Autodesk Inventor part; units mm, degrees
ref_plane "YZ Plane" through (0, 0, 0) normal (1, 0, 0) x (0, 1, 0)
ref_plane "XZ Plane" through (0, 0, 0) normal (0, 1, 0) x (-1, 0, 0)
ref_plane "XY Plane" through (0, 0, 0) normal (0, 0, 1) x (1, 0, 0)
sketch "Sketch1" plane through (0, 0, 0) normal (0, 1, 0) x (-1, 0, 0)
  line L0 (30, 30) -> (-30, 30)
  line L1 (-30, 30) -> (-30, -30)
  line L2 (-30, -30) -> (30, -30)
  line L3 (30, -30) -> (30, 30)
  line L4 (30, 30) -> (-30, -30) construction
  line L5 (-30, 30) -> (30, -30) construction
  circle A0 centre (0, 0) radius 29
  circle A1 centre (0, 0) radius 30
  point P0 (0, 0)
  dimension "d0" = 60
  dimension "d1" = 60
  dimension "d2" = 58
extrude "Extrusion1" add sketch "Sketch1" along normal blind 28 contours L3 A1 L0 | A1 L1 L0 | A1 | L3 L2 A1 | A1 L2 L1 | A0
sketch "Sketch2" plane through (0, 28, 0) normal (0, 1, 0) x (1, 0, 0)
  circle A0 centre (0, 0) radius 30
extrude "Extrusion2" add sketch "Sketch2" along normal blind 3
sketch "Sketch3" plane through (0, 31, 0) normal (0, 1, 0) x (1, 0, 0)
  circle A0 centre (0, 0) radius 29
  dimension "d7" = 58
extrude "Extrusion3" add sketch "Sketch3" along normal blind 39.5
sketch "Sketch4" plane through (0, 70.5, 0) normal (0, 1, 0) x (1, 0, 0)
  line L0 (-30, -30) -> (30, -30)
  line L1 (30, -30) -> (30, 30)
  line L2 (-30, -30) -> (30, -30)
  line L3 (30, -30) -> (30, 30)
  line L4 (30, 30) -> (-30, 30)
  line L5 (-30, 30) -> (-30, -30)
  line L6 (30, 30) -> (-30, 30) construction
  line L7 (-30, -30) -> (30, 30) construction
  line L8 (30, -30) -> (-30, 30) construction
  circle A0 centre (-23.575, -23.575) radius 2.5
  circle A1 centre (-23.575, 23.575) radius 2.5
  circle A2 centre (23.575, 23.575) radius 2.5
  circle A3 centre (23.575, -23.575) radius 2.5
  line L9 (-23.575, -23.575) -> (-23.575, 23.575) construction
  point P0 (0, 0)
  dimension "d10" = 5
  dimension "d11" = 5
  dimension "d12" = 47.15
  dimension "d13" = 5
  dimension "d14" = 5
  dimension "d15" = 47.15
  dimension "d16" = 47.15
  dimension "d17" = 47.15
sketch "Sketch5" plane through (-30, 0, 30) normal (0, 0, 1) x (1, 0, 0)
  line L0 (0, 0) -> (0, 28) construction
  line L1 (0, 70.5) -> (0, 0) construction
  line L2 (59, 70.5) -> (1, 70.5)
  point P0 (30, 0)
  dimension "d21" = 70.5
extrude "Extrusion4" add sketch "Sketch4" along normal blind 19
sketch "Sketch6" plane through (0, 89.5, 0) normal (0, 1, 0) x (1, 0, 0)
  circle A0 centre (0, 0) radius 20
  circle A1 centre (0, 0) radius 17
  circle A2 centre (0, 0) radius 7
  dimension "d22" = 14
  dimension "d23" = 40
  dimension "d24" = 3
extrude "Extrusion5" add sketch "Sketch6" along normal blind 2.5 contours A0
sketch "Sketch7" plane through (0, 89.5, 0) normal (0, 1, 0) x (1, 0, 0)
  circle A0 centre (0, 0) radius 7
  dimension "d27" = 14
extrude "Extrusion6" add sketch "Sketch7" along normal blind 35
chamfer "Chamfer1" distance 5 angle 45 8 edges at (-30, 80, 30) (30, 80, 30) (-30, 14, 30) (30, 14, 30) (30, 80, -30) (-30, 80, -30) (-30, 14, -30) (30, 14, -30)
sketch "Sketch8" plane through (0, 0, 0) normal (0, -1, 0) x (1, 0, 0)
  circle A0 centre (0, 0) radius 4
  dimension "d33" = 8
extrude "Extrusion7" cut sketch "Sketch8" against normal blind 30
equation "\"d1\" = d0"
equation "\"d15\" = d12"
equation "\"d16\" = d12"
equation "\"d17\" = d12"
properties part number "Gearbox"
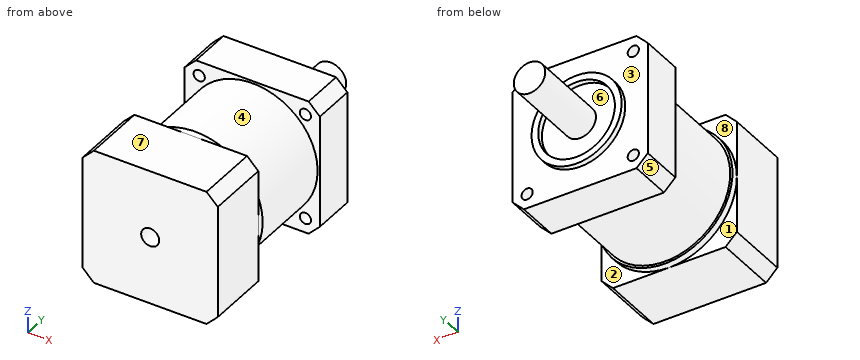
The listing builds one solid part. Answer for the finished solid, in the listing's coordinates (mm). Face numbers are marked on the shaded views. A direction names the side the tool comes from. Give positions to 0.01 mm unless a question says otherwise; leave off trailing zeros. Loops run counter-clockwise (first coordinate to the right, second up) from the corner with the lowest first, then second, coordinate; pieces in that order, holes last.
Item 1: A tool of negligible diameter and unlimited length cuts with its end or side. For the marked faces 1, 2, 3, 4 and 5, from which of +Z, -Z, +X, -X, +Y, -Y can it reach the whole face along a straight path? Write none if from no direction.
Derived:
face 1: -Z, -X
face 2: -Z, +X
face 3: +Y
face 4: none
face 5: -Z, -X, +Y, -Y
Item 2: Determine the mould class of the marked faces 6, 7 and 8 for opening direction Y: +Y half, -Y half, draft (parallel to the pull), parting line (faces both ways), or undercut.
Derived:
face 6: +Y half
face 7: draft
face 8: undercut
Item 3: A cutting plane is placed at B-B (y = 42.5). Give the vertices of the cut face in (x, z).
Derived:
outline: circle Ø58 at (0, 0)
Item 4: Each of these flat-tipped pins is pushed along its axis until it touches: pin 1 Ø6 at (x, z) = (-23.575, -23.575) entering from +Y; pin 2 Ø6.5 at (x, z) = (1, 2) entering from -Y; pin 3 Ø4 at (x, y) = (5, 38) entering from +Z; pin 4 Ø4 at (x, z) = (-23.575, 23.575) entering from +Y. Where does it stop, or does it pass through?
Derived:
pin 1: stops at y = 89.5
pin 2: stops at y = 0
pin 3: stops at z = 28.84
pin 4: stops at y = 28
Item 5: Find the intervals of material crossed by line 1 along X through (y, z) = (90.7, 0); line 2 along Y through (x, z) = (15, 27.5); line 3 along Y through (x, z) = (-24.5, -17), in increasing order.
Derived:
line 1: x = -20 to -17, -7 to 7, 17 to 20
line 2: y = 0 to 28, 70.5 to 89.5
line 3: y = 0 to 31, 70.5 to 89.5
Item 6: A cutting plane is placed at D-D (y = 96.5). Give the vertices of the cut face in (x, z), then the cut area to 3 significant figures.
Derived:
outline: circle Ø14 at (0, 0)
area: 154 mm2
Item 7: A cutting plane is placed at C-C (z = -11). Give the vertices of the cut face in (x, y).
Derived:
outline: (-30, 0) - (30, 0) - (30, 28) - (27.91, 28) - (27.91, 31) - (26.83, 31) - (26.83, 70.5) - (30, 70.5) - (30, 89.5) - (16.7, 89.5) - (16.7, 92) - (12.96, 92) - (12.96, 89.5) - (-12.96, 89.5) - (-12.96, 92) - (-16.7, 92) - (-16.7, 89.5) - (-30, 89.5) - (-30, 70.5) - (-26.83, 70.5) - (-26.83, 31) - (-27.91, 31) - (-27.91, 28) - (-30, 28) - close
